from build123d import *

# Parameters (mm, degrees)
SKETCH2_R           = 4.75
BOSS_EXTRUDE1_DEPTH = 4.5
BOSS_EXTRUDE2_DEPTH = 5.5


with BuildPart() as part:
    # Sketch2 → Boss-Extrude1 (new, symmetric)
    with BuildSketch(Plane(origin=(0, 0, 0), x_dir=(1, 0, 0), z_dir=(0, 1, 0))):
        with BuildLine():
            Line((0, 9), (88, 9))
            ThreePointArc((88, 9), (90.828427125, 7.828427125), (92, 5))
            Line((92, 5), (92, -4))
            ThreePointArc((92, -4), (87.649616471, -8.95762024), (82.168800624, -5.288220705))
            ThreePointArc((82.168800624, -5.288220705), (80.781578904, -2.951663086), (78.377159701, -1.685703406))
            Line((78.377159701, -1.685703406), (55.879764884, 3.096265482))
            ThreePointArc((55.879764884, 3.096265482), (50.580227318, 0.823270393), (50.946735477, -4.93149084))
            ThreePointArc((50.946735477, -4.93149084), (51.255135572, -7.579056787), (49, -9))
            Line((49, -9), (0, -9))
            ThreePointArc((0, -9), (-9, 0), (0, 9))
        make_face()
        with Locations(Location((0, 0, 0), (0, 0, 270))):
            Circle(SKETCH2_R, mode=Mode.SUBTRACT)
    extrude(amount=BOSS_EXTRUDE1_DEPTH, both=True)

    # Sketch2_3 → Boss-Extrude2 (add, symmetric)
    with BuildSketch(Plane(origin=(0, 0, 0), x_dir=(1, 0, 0), z_dir=(0, 1, 0))):
        with BuildLine():
            Line((0, 9), (88, 9))
            ThreePointArc((88, 9), (90.828427125, 7.828427125), (92, 5))
            Line((92, 5), (92, -4))
            ThreePointArc((92, -4), (87.649616471, -8.95762024), (82.168800624, -5.288220705))
            ThreePointArc((82.168800624, -5.288220705), (80.781578904, -2.951663086), (78.377159701, -1.685703406))
            Line((78.377159701, -1.685703406), (55.879764884, 3.096265482))
            ThreePointArc((55.879764884, 3.096265482), (50.580227318, 0.823270393), (50.946735477, -4.93149084))
            ThreePointArc((50.946735477, -4.93149084), (51.255135572, -7.579056787), (49, -9))
            Line((49, -9), (0, -9))
            ThreePointArc((0, -9), (-9, 0), (0, 9))
        make_face()
        with BuildLine():
            Line((0, 8), (88, 8))
            ThreePointArc((88, 8), (90.121320344, 7.121320344), (91, 5))
            Line((91, 5), (91, -4))
            ThreePointArc((91, -4), (87.519693176, -7.966096192), (83.135040499, -5.030576564))
            ThreePointArc((83.135040499, -5.030576564), (81.470374435, -2.226707421), (78.585071392, -0.707555806))
            Line((78.585071392, -0.707555806), (56.087676575, 4.074413083))
            ThreePointArc((56.087676575, 4.074413083), (49.728231496, 1.346818976), (50.168041286, -5.558894504))
            ThreePointArc((50.168041286, -5.558894504), (50.353081343, -7.147434072), (49, -8))
            Line((49, -8), (0, -8))
            ThreePointArc((0, -8), (-8, 0), (0, 8))
        make_face(mode=Mode.SUBTRACT)
    extrude(amount=BOSS_EXTRUDE2_DEPTH, both=True)


solid = part.part
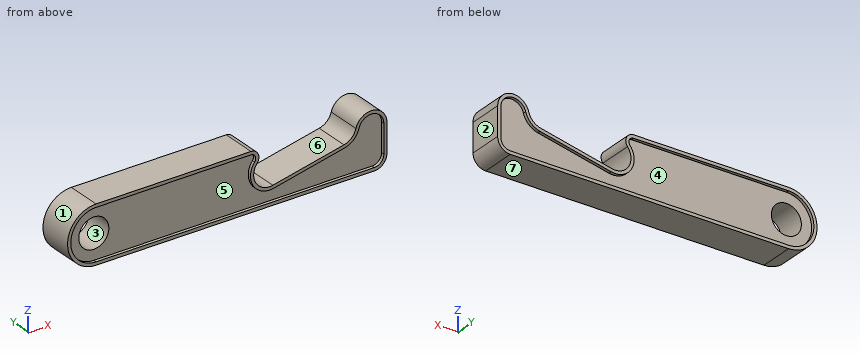
Geometry check sheet. Reference: the model listing, model coordinates, mm. Face numbers are marked on the shaded views. A direction names the side the tool comes from. Give positions to 0.01 mm unless a question says otherwise; leave off trailing zeros. Loops run counter-clockwise (first coordinate to the right, second up) from the corner with the lowest first, then second, coordinate; pieces in that order, holes last.
(1) Release check for a two-part mould opening along X. For the marked faces 1, 2, 3 and 4 record: released by +X, released by -X, zero draft, split by the parting line, or undercut.
From the geometry:
face 1: released by -X
face 2: released by +X
face 3: undercut
face 4: undercut
(2) Depth check by flat-ended pin: pin 1 Ø3 at (x, z) = (31.5, 0.5) entering from -Y; pin 2 Ø1.1 at (y, z) = (-5, -2) entering from -X; pin 3 Ø5 at (x, y) = (62, -1.5) entering from +Z. Enter the tip coordinate at first touch or a pass-through.
From the geometry:
pin 1: stops at y = -4.5
pin 2: stops at x = -8.88
pin 3: stops at z = -1.26
(3) Section check A-A on x = 20. Record the cut outline in (y, z), then the cut area to 3 significant figures.
From the geometry:
outline: (-5.5, -9) - (5.5, -9) - (5.5, -8) - (4.5, -8) - (4.5, 8) - (5.5, 8) - (5.5, 9) - (-5.5, 9) - (-5.5, 8) - (-4.5, 8) - (-4.5, -8) - (-5.5, -8) - close
area: 166 mm2
(4) Section check C-C on z = -1.5. Record the cut outline in (x, y), then the cut area to 3 significant figures.
From the geometry:
outline: (-8.87, -5.5) - (-7.86, -5.5) - (-7.86, -4.5) - (-4.51, -4.5) - (-4.51, 4.5) - (-7.86, 4.5) - (-7.86, 5.5) - (-8.87, 5.5) - close; (4.51, -4.5) - (49.83, -4.5) - (49.83, -5.5) - (51.08, -5.5) - (51.08, 5.5) - (49.83, 5.5) - (49.83, 4.5) - (4.51, 4.5) - close; (63.39, -5.5) - (68.2, -5.5) - (68.2, -4.5) - (91, -4.5) - (91, -5.5) - (92, -5.5) - (92, 5.5) - (91, 5.5) - (91, 4.5) - (68.2, 4.5) - (68.2, 5.5) - (63.39, 5.5) - close
area: 732 mm2
(5) Section check B-B on y = 0.75. Record the cut outline in (x, z).
From the geometry:
outline: (0, -9) - (88, -9) arc R4 ccw to (92, -5) - (92, 4) arc R5 ccw to (82.17, 5.29) arc R5 cw to (78.38, 1.69) - (55.88, -3.1) arc R5 cw to (50.95, 4.93) arc R2.5 ccw to (49, 9) - (0, 9) arc R9 ccw to start; hole circle Ø9.5 at (0, 0)
(6) Thickness scan on L1, parallel to X at y = 1, z = 2.25; L2, parallel to X at y = -0.25, z = 2; L3, parallel to Y at x = 45.5, z = 4.5. Record the ranges inside material, lowest first.
From the geometry:
L1: x = -8.71 to -4.18, 4.18 to 49.86, 79.84 to 92
L2: x = -8.77 to -4.31, 4.31 to 49.84, 79.35 to 92
L3: y = -4.5 to 4.5
(7) Set-up check for the marked faces 5, 6 and 7: record each of +Z, -Z, +X, -X, +Y, -Y from which the full face is reachable in a straight line by a thin tool's end or side.
From the geometry:
face 5: -Y
face 6: +Z, +Y, -Y
face 7: -Z, +X, -X, +Y, -Y
(8) Section check D-D on x = 60. Record the cut outline in (y, z), then the cut area to 3 significant figures.
From the geometry:
outline: (-5.5, -9) - (5.5, -9) - (5.5, -8) - (4.5, -8) - (4.5, -3.24) - (5.5, -3.24) - (5.5, -2.22) - (-5.5, -2.22) - (-5.5, -3.24) - (-4.5, -3.24) - (-4.5, -8) - (-5.5, -8) - close
area: 65.1 mm2
